Could you check a few things on this model? Use its own coordinates, in mm. Coordinates: 2 decimals unless noted, no trailing zeros. Write each loop counter-clockwise with the first axis right and the second up, starting at its lowest first coordinate (ties: lowest second). Pieces come first, ordered by that corner, then holes.
```python
from build123d import *

# Parameters (mm, degrees)
F0_R            = 29
F1_DEPTH        = 7
F3_DEPTH        = 12
F6_DEPTH        = 11
F6_COPIES_COUNT = 12
F9_DEPTH        = 5
F11_DEPTH       = 3.2
F13_DEPTH       = 15


# Not quite as in the source:
# - a pattern or mirror of a feature is missing from the dataset's text; its kind, count and spacing are read off the source's solid


with BuildPart() as f1:
    # F0 (on Front) → F1 (new body)
    with BuildSketch(Plane.XZ):
        Circle(F0_R)
    extrude(amount=F1_DEPTH)

    # F2 (on face) → F3 (join)
    with BuildSketch(Plane.XZ.offset(7)):
        with BuildLine():
            Line((0, -2.75), (0, 2.75))
            ThreePointArc((0, 2.75), (-0.7424621202, 3.0575378798), (-1.05, 3.8))
            Line((-1.05, 3.8), (-1.05, 4.6324939288))
            ThreePointArc((-1.05, 4.6324939288), (-4.75, 0), (-1.05, -4.6324939288))
            Line((-1.05, -4.6324939288), (-1.05, -3.8))
            ThreePointArc((-1.05, -3.8), (-0.7424621202, -3.0575378798), (0, -2.75))
        make_face()
        with BuildLine():
            ThreePointArc((1.05, -4.6324939288), (3.711468712, -2.9643717716), (4.75, 0))
            ThreePointArc((4.75, 0), (3.711468712, 2.9643717716), (1.05, 4.6324939288))
            Line((1.05, 4.6324939288), (1.05, 3.8))
            ThreePointArc((1.05, 3.8), (0.7424621202, 3.0575378798), (0, 2.75))
            Line((0, 2.75), (0, -2.75))
            ThreePointArc((0, -2.75), (0.7424621202, -3.0575378798), (1.05, -3.8))
            Line((1.05, -3.8), (1.05, -4.6324939288))
        make_face()
    extrude(amount=F3_DEPTH)

    # F5 (on offset) → F6 (cut)
    with BuildSketch(Plane.YZ.offset(29)):
        Polygon((-2.8396848584, -1.3322586236), (-1.4665255865, -2.8938910614), (0.5622881169, -3.3501554734), (2.4718183739, -2.5267743623), (3.5326895289, -0.7382513266), (3.3396848584, 1.3322586236), (1.9665255865, 2.8938910614), (-0.0622881169, 3.3501554734), (-1.9718183739, 2.5267743623), (-3.0326895289, 0.7382513266), align=None)
    f6 = extrude(amount=-F6_DEPTH, mode=Mode.SUBTRACT)

    # F6_copies: F6 ×12 about axis
    f6_copies_axis = Axis((0, 0, 0), (0, 1, 0))
    for i in range(1, F6_COPIES_COUNT):
        add(f6.rotate(f6_copies_axis, i * 360 / F6_COPIES_COUNT), mode=Mode.SUBTRACT)

    # F8 (on face) → F9 (join)
    with BuildSketch(Plane.XZ.offset(7)):
        Polygon((8.2854374709, 4.7012260014), (0.0713375892, 9.5260123319), (-8.2140998816, 4.8247863305), (-0.0713375892, -9.5260123319), (8.2140998816, -4.8247863305), align=None)
        with BuildLine():
            ThreePointArc((-1.05, -4.6324939288), (-4.75, 0), (-1.05, 4.6324939288))
            Line((-1.05, 4.6324939288), (-1.05, 3.8))
            ThreePointArc((-1.05, 3.8), (0, 2.75), (1.05, 3.8))
            Line((1.05, 3.8), (1.05, 4.6324939288))
            ThreePointArc((1.05, 4.6324939288), (4.75, 0), (1.05, -4.6324939288))
            Line((1.05, -4.6324939288), (1.05, -3.8))
            ThreePointArc((1.05, -3.8), (0, -2.75), (-1.05, -3.8))
            Line((-1.05, -3.8), (-1.05, -4.6324939288))
        make_face(mode=Mode.SUBTRACT)
        with BuildLine():
            Line((-1.05, 3.8), (-1.05, 4.6324939288))
            ThreePointArc((-1.05, 4.6324939288), (-4.75, 0), (-1.05, -4.6324939288))
            Line((-1.05, -4.6324939288), (-1.05, -3.8))
            ThreePointArc((-1.05, -3.8), (0, -2.75), (1.05, -3.8))
            Line((1.05, -3.8), (1.05, -4.6324939288))
            ThreePointArc((1.05, -4.6324939288), (4.75, 0), (1.05, 4.6324939288))
            Line((1.05, 4.6324939288), (1.05, 3.8))
            ThreePointArc((1.05, 3.8), (0, 2.75), (-1.05, 3.8))
        make_face()
    extrude(amount=F9_DEPTH)

    # F10 (on face) → F11 (cut)
    with BuildSketch(Plane.XZ.offset(7)):
        Polygon((4.92104771, 2.7922433221), (0.0423702045, 5.6578739911), (-4.8786775054, 2.865630669), (-4.92104771, -2.7922433221), (-0.0423702045, -5.6578739911), (4.8786775054, -2.865630669), align=None)
        Polygon((-4.92104771, -2.7922433221), (-4.8786775054, 2.865630669), (-9.9290630252, 0), (-5.0927557243, -8.5235046601), (-0.0423702045, -5.6578739911), align=None)
    extrude(amount=F11_DEPTH, mode=Mode.SUBTRACT)

    # F12 (on face) → F13 (cut)
    with BuildSketch(Plane(origin=(0, 0, 0), x_dir=(-1, 0, 0), z_dir=(0, 1, 0))):
        Polygon((2.9053820181, 0.8348685994), (1.8597799775, 2.3831635875), (0.103805197, 3.0211710859), (-1.6918196405, 2.5051939154), (-2.8412268781, 1.0323178175), (-2.9053820181, -0.8348685994), (-1.8597799775, -2.3831635875), (-0.103805197, -3.0211710859), (1.6918196405, -2.5051939154), (2.8412268781, -1.0323178175), align=None)
    extrude(amount=-F13_DEPTH, mode=Mode.SUBTRACT)


solid = f1.part
```
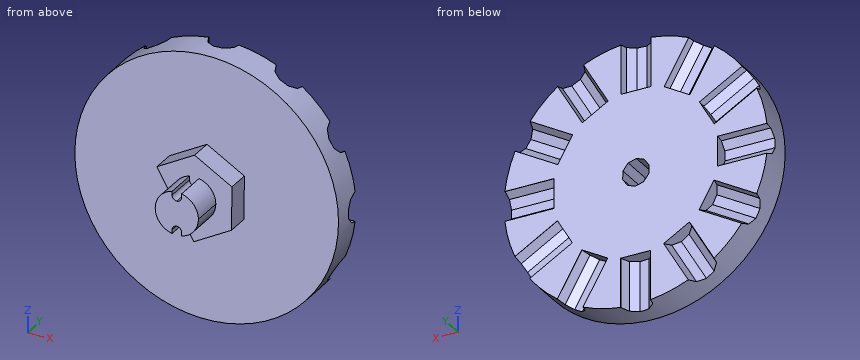
Item 1: If I drill on line 1 along X through (y, z) = (-2.5, -20); line 2 along Z through (x, y) = (-16.5, -2.75); line 3 along Z through (x, y) = (0, -17.5), over which ranges is the centre line in solid material (lowest first)?
Item 2: I want a section at A-A, the plane z = -20. List the corners of the cut face in (x, y) for me, then the cut area to 3 significant figures.
Item 3: Will these pins go through, and if not, where does the flat tip stop? pin 1 Ø0.7 at (y, z) = (-15, 4.5) entering from -X; pin 2 Ø1.5 at (y, z) = (-1.5, -1.5) entering from -X; pin 3 Ø10 at (y, z) = (-4, -23) entering from +X.
Item 4: I want a section at B-B, the plane x = 22. List the corners of the cut face in (y, z) for me.
Taken from the geometry:
1. line 1: x = -21 to -13.53, -9.66 to -1.72, 1.64 to 9.56, 13.44 to 21
1. line 2: z = -23.85 to -10.93, -7.87 to 8.12, 11.18 to 23.85
1. line 3: z = -2.75 to 2.75
2. outline: (-21, -7) - (21, -7) - (21, 0) - (15.4, 0) - (15.42, -0.06) - (14.46, -1.97) - (12.4, -3.03) - (10.01, -2.84) - (8.21, -1.47) - (7.82, 0) - (3.34, 0) - (3.35, -0.06) - (2.53, -1.97) - (0.74, -3.03) - (-1.33, -2.84) - (-2.89, -1.47) - (-3.22, 0) - (-7.69, 0) - (-7.68, -0.06) - (-8.63, -1.97) - (-10.69, -3.03) - (-13.09, -2.84) - (-14.89, -1.47) - (-15.27, 0) - (-21, 0) - close
2. area: 244 mm2
3. pin 1: stops at x = -2.31
3. pin 2: stops at x = -18
3. pin 3: stops at x = 22.74
4. outline: (-7, -18.89) - (0, -18.89) - (0, -16.42) - (-1.47, -16.04) - (-2.84, -14.24) - (-3.03, -11.85) - (-1.97, -9.78) - (-0.06, -8.83) - (0, -8.85) - (0, -3.22) - (-1.47, -2.89) - (-2.84, -1.33) - (-3.03, 0.74) - (-1.97, 2.53) - (-0.06, 3.35) - (0, 3.34) - (0, 8.98) - (-1.47, 9.36) - (-2.84, 11.16) - (-3.03, 13.55) - (-1.97, 15.62) - (-0.06, 16.57) - (0, 16.55) - (0, 18.89) - (-7, 18.89) - close
